Check sheet for the modelled part. Datum: model origin and axes. Units: mm. Give positions to 0.01 mm unless a question says otherwise; leave off trailing zeros.
```python
from build123d import *

# Parameters (mm, degrees)
SKETCH1_R           = 2
BOSS_EXTRUDE2_DEPTH = 10
FILLET4_R           = 2
FILLET5_R           = 2


with BuildPart() as part:
    # Sketch1 → Boss-Extrude2 (new body)
    with BuildSketch(Plane.XY):
        with BuildLine():
            ThreePointArc((47.515201165, 28.636720293), (51.481242597, 23.445158013), (47.04657628, 18.647706792))
            add(Edge.make_bspline(
                [(47.04657628, 18.647706792), (23.149465596, 14.415740026), (22.411661364, 8.636217355)],
                knots=[0, 0, 0, 0.485397068, 0.485397068, 0.485397068], degree=2))
            add(Edge.make_bspline(
                [(47.04657628, -1.374266206), (23.149465596, 2.856694684), (22.411661364, 8.636217355)],
                knots=[0, 0, 0, 0.485397068, 0.485397068, 0.485397068], degree=2))
            ThreePointArc((47.04657628, -1.374266206), (52.04657628, -6.145195345), (47.515201165, -11.363279707))
            add(Edge.make_bspline(
                [(47.515201165, -11.363279707), (10.933254614, -0.926951504), (10.411661364, 8.636217355)],
                knots=[0, 0, 0, 0.478869132, 0.478869132, 0.478869132], degree=2))
            add(Edge.make_bspline(
                [(47.515201165, 28.636720293), (10.933254614, 18.199386214), (10.411661364, 8.636217355)],
                knots=[0, 0, 0, 0.478869132, 0.478869132, 0.478869132], degree=2))
        make_face()
        with Locations((47.04657628, -6.379765498)):
            Circle(SKETCH1_R, mode=Mode.SUBTRACT)
    extrude(amount=BOSS_EXTRUDE2_DEPTH)

    # Fillet4
    fillet4_edges = [part.edges().sort_by_distance(p)[0] for p in [
        (47.515201165, 28.636720293, 5),
    ]]
    fillet(fillet4_edges, radius=FILLET4_R)

    # Fillet5
    fillet5_edges = [part.edges().sort_by_distance(p)[0] for p in [
        (47.515201165, -11.363279707, 5),
    ]]
    fillet(fillet5_edges, radius=FILLET5_R)


solid = part.part
```
(1) Gauge pin test, flat ends, axial feed: pin 1 Ø1 at (x, z) = (35, 3.5) entering from +Y; pin 2 Ø1 at (x, z) = (41, 8) entering from +Y; pin 3 Ø4 at (x, z) = (41.5, 5.5) entering from +Y; pin 4 Ø5 at (x, y) = (44.5, 3.5) entering from +Z. Record the tip position at first contact, or that the pin passes through.
Response values:
pin 1: stops at y = 24.9
pin 2: stops at y = 26.85
pin 3: stops at y = 27.46
pin 4: passes through
(2) Release check for a two-part mould opening along Y. For faces 1 (the face through (26.9, 13.3, 10)), 2 (the face through (45.05, -6.29, 4.93)) record: released by +Y, released by -Y, zero draft, split by the parting line, or undercut.
Response values:
face 1: zero draft
face 2: undercut
(3) Material ranges on L1, parallel to Y at x = 48.5, z = 7.5; L2, parallel to Y at x = 47, z = 0.75; L3, parallel to Y at x = 29, z = 1, recorded low to high.
Response values:
L1: y = -11.17 to -7.75, -5.01 to -1.59, 19.06 to 28.31
L2: y = -11.22 to -8.38, -4.38 to -1.37, 18.64 to 28.49
L3: y = -5.25 to 3.22, 14.05 to 22.53
